```python
from build123d import *

# Parameters (mm, degrees)
BOSS_EXTRUDE1_DEPTH = 12
SKETCH2_R           = 1.55
CUT_EXTRUDE1_DEPTH  = 23.135943621
CUT_EXTRUDE2_DEPTH  = 1.5
SKETCH4_R           = 1.55
CUT_EXTRUDE3_DEPTH  = 23.135943621
CUT_EXTRUDE4_DEPTH  = 1.5
FILLET1_R           = 2
FILLET2_R           = 1
FILLET3_R           = 3


with BuildPart() as part:
    # Sketch1 → Boss-Extrude1 (new body)
    with BuildSketch(Plane.XY):
        Polygon((0, 0), (0, 15), (4, 15), (4, 4), (15, 4), (15, 0), align=None)
    extrude(amount=BOSS_EXTRUDE1_DEPTH)

    # Sketch2 → Cut-Extrude1 (cut, through all)
    with BuildSketch(Plane(origin=(0, 4, 0), x_dir=(1, 0, 0), z_dir=(0, 1, 0))):
        with Locations(Location((9, -6, 0), (0, 0, 270))):
            Circle(SKETCH2_R)
    extrude(amount=-CUT_EXTRUDE1_DEPTH, mode=Mode.SUBTRACT)

    # Sketch3 → Cut-Extrude2 (cut)
    with BuildSketch(Plane(origin=(0, 4, 0), x_dir=(1, 0, 0), z_dir=(0, 1, 0))):
        Polygon((5.478163358, -6), (7.239081679, -9.05), (10.760918321, -9.05), (12.521836642, -6), (10.760918321, -2.95), (7.239081679, -2.95), align=None)
    extrude(amount=-CUT_EXTRUDE2_DEPTH, mode=Mode.SUBTRACT)

    # Sketch4 → Cut-Extrude3 (cut, through all)
    with BuildSketch(Plane(origin=(4, 0, 0), x_dir=(0, 0, -1), z_dir=(1, 0, 0))):
        with Locations(Location((-6, 9, 0), (0, 0, 90))):
            Circle(SKETCH4_R)
    extrude(amount=-CUT_EXTRUDE3_DEPTH, mode=Mode.SUBTRACT)

    # Sketch5 → Cut-Extrude4 (cut)
    with BuildSketch(Plane(origin=(4, 0, 0), x_dir=(0, 0, -1), z_dir=(1, 0, 0))):
        Polygon((-6, 5.478163358), (-2.95, 7.239081679), (-2.95, 10.760918321), (-6, 12.521836642), (-9.05, 10.760918321), (-9.05, 7.239081679), align=None)
    extrude(amount=-CUT_EXTRUDE4_DEPTH, mode=Mode.SUBTRACT)

    # Fillet1
    fillet1_edges = [part.edges().sort_by_distance(p)[0] for p in [
        (0, 7.45, 6),
    ]]
    fillet(fillet1_edges, radius=FILLET1_R)

    # Fillet2
    fillet2_edges = [part.edges().sort_by_distance(p)[0] for p in [
        (4, 4, 6),
    ]]
    fillet(fillet2_edges, radius=FILLET2_R)

    # Fillet3
    fillet3_edges = [part.edges().sort_by_distance(p)[0] for p in [
        (2, 15, 12),
        (2, 15, 0),
        (15, 2, 12),
        (15, 2, 0),
    ]]
    fillet(fillet3_edges, radius=FILLET3_R)


solid = part.part
```
Verification items for the finished model (mm, model axes). A direction names the side the tool comes from. Coordinates: 2 decimals unless noted, no trailing zeros. Write each loop counter-clockwise with the first axis right and the second up, starting at its lowest first coordinate (ties: lowest second). Pieces come first, ordered by that corner, then holes. Notation, with made-up numbers: M 71.5,-7 L 119.5,-7 A21 ccw 119.5,0 Z; hole C -19.5,28 d5. An arc over 180 degrees is marked long. Answer as a JSON object with one key per item and string values. Group by question number.
(1) Gauge pin test, flat ends, axial feed: pin 1 (4 mm diameter, centred on y = 9.5, z = 9, fed in from +X); pin 2 (3 mm diameter, centred on x = 12, z = 1.5, fed in from -Y); pin 3 (8 mm diameter, centred on x = 10.5, y = 11, fed in from -Z); pin 4 (5 mm diameter, centred on x = 8.5, z = 6, fed in from +Y). Record the tip position at first contact, or that the pin passes through.
(2) Release check for a two-part mould opening along Z. For faces 5 (the face through (12.2, 4, 4.6)), 6 (the face through (2.5, 7, 7)), 7 (the face through (2.03, 14.1, 0.86)) record: +Z half, -Z half, draft (parallel to the pull), parting line (faces both ways), or undercut.
(3) Cross-section at C-C, the plane y = 9. Record the cut outline in (x, z).
(4) Tool access check on faces 1 (the face through (3.26, 6.371, 7.546)), 2 (the face through (11.654, 3.26, 4.496)), 3 (the face through (15, 2, 6)), 4 (the face through (4, 12.3, 4.6)). Record the directions out of +Z, -Z, +X, -X, +Y, -Y that give a thin tool (end or side, any length) a straight path to the whole face; none if there is none.
(5) Cross-section at B-B, the plane x = 9. Record the cut outline in (y, z), and give its area (3 significant figures).
(6) Cross-section at A-A, the plane y = 2. Record the cut outline in (x, z).
(7) Material ranges on line 1 (Z direction, x = 2.1, y = 9); line 2 (X direction, y = 0.75, z = 6); line 3 (Z direction, x = 8.5, y = 3.75), recorded low to high.
(8) Cross-section at D-D, the plane x = 1.25. Record the cut outline in (y, z).
Reply:
{
 "1": {"pin 1": "x = 4", "pin 2": "y = 0", "pin 3": "through", "pin 4": "y = 2.5"},
 "2": {"face 5": "draft", "face 6": "undercut", "face 7": "-Z half"},
 "3": {"outline": "M 0,0 L 4,0 L 4,2.95 L 2.5,2.95 L 2.5,4.45 L 2,4.45 A2 ccw 0,2.45 Z; M 0,9.55 A2 ccw 2,7.55 L 2.5,7.55 L 2.5,9.05 L 4,9.05 L 4,12 L 0,12 Z"},
 "4": {"face 1": "+X", "face 2": "+Y", "face 3": "+Z, -Z, +X, +Y, -Y", "face 4": "+Z, -Z, +X, +Y"},
 "5": {"outline": "M 0,0 L 4,0 L 4,2.95 L 2.5,2.95 L 2.5,4.45 L 0,4.45 Z; M 0,7.55 L 2.5,7.55 L 2.5,9.05 L 4,9.05 L 4,12 L 0,12 Z", "area": "31.1 mm²"},
 "6": {"outline": "M 0,0 L 12,0 A3 ccw 15,3 L 15,9 A3 ccw 12,12 L 0,12 Z; hole C 9,6 d3.1"},
 "7": {"line 1": "0 to 4.45, 7.55 to 12", "line 2": "0 to 7.45, 10.55 to 15", "line 3": "0 to 2.95, 9.05 to 12"},
 "8": {"outline": "M 0,0 L 12,0 A3 ccw 15,3 L 15,9 A3 ccw 12,12 L 0,12 Z; hole C 9,6 d3.39"}
}
